from build123d import *

# Parameters (mm, degrees)
BOSS_EXTRUDE1_DEPTH = 9.525


with BuildPart() as part:
    # Sketch1 → Boss-Extrude1 (new body)
    with BuildSketch(Plane(origin=(0, 0, 0), x_dir=(1, 0, 0), z_dir=(0, 1, 0))):
        with BuildLine():
            Line((-46.373035196, 23.110309708), (-64.906111076, 36.564296932))
            ThreePointArc((-64.906111076, 36.564296932), (-66.328511848, 36.789669498), (-67.347825731, 35.772312158))
            Line((-67.347825731, 35.772312158), (-75.28680268, 11.455483186))
            ThreePointArc((-75.28680268, 11.455483186), (-75.067914414, 10.037862192), (-73.795636305, 9.375389727))
            Line((-73.795636305, 9.375389727), (-50.87703604, 9.116346342))
            ThreePointArc((-50.87703604, 9.116346342), (-49.759830806, 8.638721158), (-49.307579416, 7.511005754))
            Line((-49.307579416, 7.511005754), (-49.484846196, -8.172492476))
            ThreePointArc((-49.484846196, -8.172492476), (-49.032594805, -9.30020788), (-47.915389571, -9.777833064))
            Line((-47.915389571, -9.777833064), (-15.849937724, -10.140261096))
            ThreePointArc((-15.849937724, -10.140261096), (-11.615281586, -10.76526167), (-7.701553332, -12.498948344))
            ThreePointArc((-7.701553332, -12.498948344), (13.937693435, -4.612844582), (1.275661223, 14.625673382))
            ThreePointArc((1.275661223, 14.625673382), (-2.899601677, 15.569134056), (-6.671010295, 17.593835357))
            Line((-6.671010295, 17.593835357), (-32.724313124, 36.507091078))
            ThreePointArc((-32.724313124, 36.507091078), (-33.90587286, 36.790269364), (-34.941599049, 36.155017749))
            Line((-34.941599049, 36.155017749), (-44.155749271, 23.462383037))
            ThreePointArc((-44.155749271, 23.462383037), (-45.19147546, 22.827131422), (-46.373035196, 23.110309708))
        make_face()
    extrude(amount=-BOSS_EXTRUDE1_DEPTH)


solid = part.part
Verification items for the finished model (mm, model axes). A direction names the side the tool comes from. Give positions to 0.01 mm unless a question says otherwise; leave off trailing zeros. Write each loop counter-clockwise with the first axis right and the second up, starting at its lowest first coordinate (ties: lowest second). Pieces come first, ordered by that corner, then holes.
(1) Gauge pin test, flat ends, axial feed: pin 1 (1 mm diameter, centred on x = -41.5, y = -7.5, fed in from +Z); pin 2 (2 mm diameter, centred on y = -4.5, z = -21.5, fed in from +X); pin 3 (3 mm diameter, centred on x = -38, z = 9.5, fed in from +Y); pin 4 (1.5 mm diameter, centred on y = -1, z = -31, fed in from -X). Record the tip position at first contact, or that the pin passes through.
(2) Access from +Z, -Z, +X, -X, +Y, -Y to the whole of each face (thin tool, end or side, straight path). Record for faces 1 (the face through (-49.77, -4.7, -8.65)), 2 (the face through (-39.48, -4.7, -29.9)), 3 (the face through (-19.52, -4.7, -26.92)).
(3) Cross-section at B-B (z = -30). Enter the section's corners in (x, y) (3 decimals), plus the area to 3 significant figures.
(4) Material ranges on line 1 (X direction, y = -4.25, z = -32); line 2 (X direction, y = -1, z = -31); line 3 (Z direction, x = -34, y = -6.5), recorded low to high.
(5) Cross-section at D-D (z = -2). Enter the section's corners in (x, y) (3 decimals), plus the area to 3 significant figures.
(6) Mould release check, pull along X, two halves, no side actions. Record for faces 4 (the face through (-75.08, -4.696, -10.055)), 5 (the face through (13.82, -4.7, 4.96)), 6 (the face through (-55.51, -4.696, -29.743)): +X half, -X half, draft (parallel to the pull), parting line (faces both ways), or undercut.
(7) Cross-section at C-C (x = -61.5). Enter the section's corners in (y, z) (3 decimals).
Worked out:
1. pin 1: stops at z = 9.86
1. pin 2: stops at x = -10.67
1. pin 3: stops at y = 0
1. pin 4: stops at x = -69.15
2. face 1: -X, +Y, -Y
2. face 2: -Z, +Y, -Y
2. face 3: -Z, +X, +Y, -Y
3. outline: (-69.232, -9.525) - (-55.864, -9.525) - (-55.864, 0) - (-69.232, 0) - close; (-39.41, -9.525) - (-23.761, -9.525) - (-23.761, 0) - (-39.41, 0) - close
3. area: 276 mm2
4. line 1: x = -68.58 to -58.62, -37.96 to -26.52
4. line 2: x = -68.91 to -57.24, -38.68 to -25.14
4. line 3: z = -36.77 to 9.94
5. outline: (-49.37, -9.525) - (14.544, -9.525) - (14.544, 0) - (-49.37, 0) - close
5. area: 609 mm2
6. face 4: -X half
6. face 5: parting line
6. face 6: undercut
7. outline: (-9.525, -34.092) - (0, -34.092) - (0, -9.236) - (-9.525, -9.236) - close
